Read the model definition and answer for the solid it produces. Units are mm, in the model's axes. A direction names the side the tool comes from. Give positions to 0.01 mm unless a question says otherwise; leave off trailing zeros. Write each loop counter-clockwise with the first axis right and the second up, starting at its lowest first coordinate (ties: lowest second). Pieces come first, ordered by that corner, then holes. Notation, with made-up numbers: M -24,-1 L -19,-1 A32 cw -19,36 Z; hole C 80.5,19.25 d2. An arc over 180 degrees is marked long. Put each result on its own line as item: value.
from build123d import *

# Parameters (mm, degrees)
SKETCH_1_W          = 250
SKETCH_1_H          = 150
EXTRUDE_1_DEPTH     = 100
SKETCH_2_R          = 25
EXTRUDE_2_DEPTH     = 0.4
SKETCH_5_W          = 245
SKETCH_5_H          = 140
CUT_EXTRUDE_1_DEPTH = 95
SKETCH_7_W          = 10
SKETCH_7_H          = 10
CUT_EXTRUDE_2_DEPTH = 5
CUT_EXTRUDE_3_DEPTH = 5
SKETCH_10_W         = 10
SKETCH_10_H         = 10
CUT_EXTRUDE_4_DEPTH = 5
CUT_EXTRUDE_6_DEPTH = 5


with BuildPart() as part:
    # 草图1 → 凸台-拉伸1 (new body)
    with BuildSketch(Plane(origin=(0, 0, 0), x_dir=(1, 0, 0), z_dir=(0, 1, 0))):
        with Locations((1.420454545, -10.84280303)):
            Rectangle(SKETCH_1_W, SKETCH_1_H)
    extrude(amount=EXTRUDE_1_DEPTH)

    # 草图2 → 凸台-拉伸2 (add)
    with BuildSketch(Plane(origin=(0, 100, 0), x_dir=(1, 0, 0), z_dir=(0, 1, 0))):
        with Locations(Location((76.420454545, -10.84280303, 0), (0, 0, 270))):
            Circle(SKETCH_2_R)
        with Locations(Location((-73.579545455, -10.84280303, 0), (0, 0, 270))):
            Circle(SKETCH_2_R)
    extrude(amount=EXTRUDE_2_DEPTH)

    # 草图5 → 切除-拉伸1 (cut)
    with BuildSketch(Plane.XZ):
        with Locations((-1.079545455, 10.84280303)):
            Rectangle(SKETCH_5_W, SKETCH_5_H)
    extrude(amount=-CUT_EXTRUDE_1_DEPTH, mode=Mode.SUBTRACT)

    # 草图7 → 切除-拉伸2 (cut)
    with BuildSketch(Plane.XY.offset(85.84280303)):
        with Locations((-118.579545455, 50)):
            Rectangle(SKETCH_7_W, SKETCH_7_H)
    extrude(amount=-CUT_EXTRUDE_2_DEPTH, mode=Mode.SUBTRACT)

    # 草图9 → 切除-拉伸3 (cut)
    with BuildSketch(Plane.XY.offset(85.84280303)):
        Polygon((-123.579545455, 55), (-113.579545455, 65), (-113.579545455, 55), align=None)
        Polygon((-123.579545455, 45), (-113.579545455, 45), (-113.579545455, 35), align=None)
    extrude(amount=-CUT_EXTRUDE_3_DEPTH, mode=Mode.SUBTRACT)

    # 草图10 → 切除-拉伸4 (cut)
    with BuildSketch(Plane(origin=(0, 0, -64.15719697), x_dir=(-1, 0, 0), z_dir=(0, 0, -1))):
        with Locations((118.579545455, 50)):
            Rectangle(SKETCH_10_W, SKETCH_10_H)
    extrude(amount=-CUT_EXTRUDE_4_DEPTH, mode=Mode.SUBTRACT)

    # 草图17 → 切除-拉伸6 (cut)
    with BuildSketch(Plane(origin=(0, 0, -64.15719697), x_dir=(-1, 0, 0), z_dir=(0, 0, -1))):
        Polygon((123.579545455, 55), (113.579545455, 65), (113.579545455, 55), align=None)
        Polygon((123.579545455, 45), (113.579545455, 35), (113.579545455, 45), align=None)
    extrude(amount=-CUT_EXTRUDE_6_DEPTH, mode=Mode.SUBTRACT)


solid = part.part
(1) Which of the six approach directions +Z, -Z, +X, -X, +Y, -Y give full straight-line access (tool end or side, diameter ignored) to faces 4 (the face through (83.93, 100.2, 34.69)), 5 (the face through (-123.58, 97, 11)), 6 (the face through (121.42, 47, 10))?
Result:
face 4: +Y
face 5: +Z, -Z, -X, +Y, -Y
face 6: -X, -Y
(2) Section D-D on x = 64 is taken. Determine the outline of the cut face in (y, z).
Result:
outline: M 0,-64.16 L 100,-64.16 L 100,-10.85 L 100.4,-10.85 L 100.4,32.54 L 100,32.54 L 100,85.84 L 0,85.84 L 0,80.84 L 95,80.84 L 95,-59.16 L 0,-59.16 Z
(3) Section A-A on z = -32 is taken. Determine the outline of the cut face in (x, y).
Result:
outline: M -123.58,95 L 121.42,95 L 121.42,0 L 126.42,0 L 126.42,100 L -123.58,100 Z
(4) Straight lines are drawn through the part: line 1 along Z through (x, y) = (111, 68.5); line 2 along X through (y, z) = (83, -23); line 3 along Y through (x, z) = (38, -14). For each, find the intervals that lie inside material, in ascending order. Write a range as from..to.
Result:
line 1: z = -64.16..-59.16, 80.84..85.84
line 2: x = 121.42..126.42
line 3: y = 95..100
(5) Given pin 1 Ø3 at (y, z) = (18, 21.5) entering from -X; pin 2 Ø1 at (x, z) = (-40.5, 64) entering from +Y; pin 3 Ø12 at (x, z) = (-92.5, 3) entering from -Y, each flat-ended and moving along its own axis, determine where each tip first touches the part or whether it passes through.
Result:
pin 1: stops at x = 121.42
pin 2: stops at y = 100
pin 3: stops at y = 95
(6) Section C-C on x = 23 is taken. Determine the outline of the cut face in (y, z), and give its area (3 significant figures).
Result:
outline: M 0,-64.16 L 100,-64.16 L 100,85.84 L 0,85.84 L 0,80.84 L 95,80.84 L 95,-59.16 L 0,-59.16 Z
area: 1,700 mm²
(7) For a pull along X with two mould halves and no side action, classify faces 1 (the face through (-123.58, 22, 83)), 2 (the face through (-113.58, 50, -62)), 3 (the face through (126.42, 49, 12)) as +X half, -X half, draft (parallel to the pull), parting line (faces both ways), or undercut.
Result:
face 1: -X half
face 2: undercut
face 3: +X half
(8) Section B-B on y = 14.5 is taken. Determine the outline of the cut face in (x, z), and give its area (3 significant figures).
Result:
outline: M -123.58,-64.16 L 126.42,-64.16 L 126.42,85.84 L -123.58,85.84 L -123.58,80.84 L 121.42,80.84 L 121.42,-59.16 L -123.58,-59.16 Z
area: 3,200 mm²
